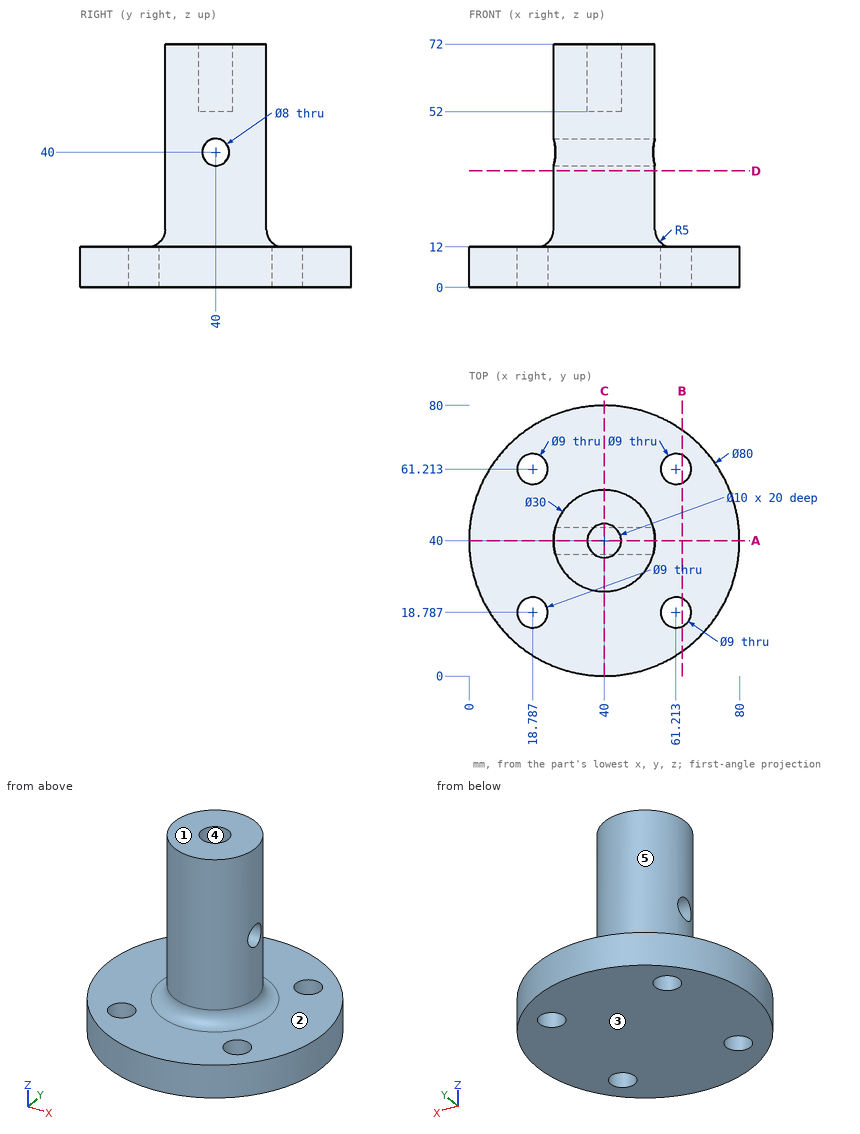
The figure shows three views and two pictorial views of one solid part (mm, origin at its lowest corner). Answer the questions. A direction names the side the tool comes from. Give positions to 0.01 mm unless a question says otherwise; leave off trailing zeros. Order: outer loops, then holes, each group sorted by start corner. A loop starts at its lowest first (then second) coordinate and runs counter-clockwise, first axis right, second up. Notation, with made-up numbers: (24.25, 4) -> (64.25, 4) arc R21 ccw to (64.25, 11) -> close; hole circle Ø10 at (89.25, 52.5). An arc over 180 degrees is marked (long way). Answer as a JSON object with one key per item and string values. Group by question number.
Item 1: The part is cut by section C-C on x = 40. Write down the section's boundary in (y, z), and give its area (3 significant figures).
Item 2: Determine the mould class of the marked faces 3, 4 and 5 for opening direction Y: pulls with the +Y half, pulls with the -Y half, needs draft (parallel to the pull), parting line crosses it, or undercut.
Item 3: Flat-ended cylindrical pins translate along their axes: pin 1 (11.5 mm diameter, centred on x = 18.79, y = 61.21, fed in from +Z); pin 2 (4 mm diameter, centred on x = 55, z = 23, fed in from -Y); pin 3 (4 mm diameter, centred on x = 46.5, z = 52, fed in from -Y). Find the tip coordinate at first contact, or state that the pin passes through.
Item 4: The part is cut by section D-D on z = 34.5. Write down the section's boundary in (x, y), and give its area (3 significant figures).
Item 5: The part is cut by section B-B on x = 63. Write down the section's boundary in (y, z), and give its area (3 significant figures).
Item 6: Consider L1, parallel to X at y = 62, z = 5.5; L2, parallel to Z at x = 42, y = 13; L3, parallel to Y at x = 49.5, z = 41.5. Determine where each line is inside the solid, lowest interval first. Write a range as from..to.
Item 7: A tool of negligible diameter and unlimited length cuts with its end or side. For the marked faces 1 and 2, from which of +Z, -Z, +X, -X, +Y, -Y can it reach the whole face along a straight path? Write none if from no direction.
Item 8: The part is cut by section A-A on y = 40. Write down the section's boundary in (x, z), and give its area (3 significant figures).
Result set:
{
 "1": {"outline": "(0, 0) -> (80, 0) -> (80, 12) -> (60, 12) arc R5 cw to (55, 17) -> (55, 72) -> (45, 72) -> (45, 52) -> (35, 52) -> (35, 72) -> (25, 72) -> (25, 17) arc R5 cw to (20, 12) -> (0, 12) -> close; hole circle Ø8 at (40, 40)", "area": "2,520 mm²"},
 "2": {"face 3": "needs draft", "face 4": "undercut", "face 5": "parting line crosses it"},
 "3": {"pin 1": "z = 12", "pin 2": "y = 32.52", "pin 3": "y = 25.69"},
 "4": {"outline": "circle Ø30 at (40, 40)", "area": "707 mm²"},
 "5": {"outline": "(7.27, 0) -> (14.66, 0) -> (14.66, 12) -> (7.27, 12) -> close; (22.92, 0) -> (57.08, 0) -> (57.08, 12) -> (22.92, 12) -> close; (65.34, 0) -> (72.73, 0) -> (72.73, 12) -> (65.34, 12) -> close", "area": "587 mm²"},
 "6": {"L1": "6.59..14.36, 23.22..56.78, 65.64..73.41", "L2": "0..12", "L3": "28.39..36.29, 43.71..51.61"},
 "7": {"face 1": "+Z, +X, -X, +Y, -Y", "face 2": "+Z"},
 "8": {"outline": "(0, 0) -> (80, 0) -> (80, 12) -> (60, 12) arc R5 cw to (55, 17) -> (55, 36) -> (25, 36) -> (25, 17) arc R5 cw to (20, 12) -> (0, 12) -> close; (25, 44) -> (55, 44) -> (55, 72) -> (45, 72) -> (45, 52) -> (35, 52) -> (35, 72) -> (25, 72) -> close", "area": "2,330 mm²"}
}
